from build123d import *

# Parameters (mm, degrees)
PAD_DEPTH       = 3
SKETCH001_R     = 2.125
POCKET_DEPTH    = 2.15
CHAMFER_SIZE    = 0.2
CHAMFER001_SIZE = 0.2


with BuildPart() as part:
    # Sketch → Pad (new body)
    with BuildSketch(Plane.XY):
        Polygon((4.618802, 0), (2.309401, 4), (-2.309401, 4), (-4.618802, 0), (-2.309401, -4), (2.309401, -4), (4.618802, -8), (9.237604, -8), (11.547005, -4), (9.237604, 0), align=None)
    extrude(amount=PAD_DEPTH)

    # Sketch001 → Pocket (cut)
    with BuildSketch(Plane.XY):
        Circle(SKETCH001_R)
    extrude(amount=POCKET_DEPTH, mode=Mode.SUBTRACT)

    # Chamfer
    chamfer_edges = [part.edges().sort_by_distance(p)[0] for p in [
        (3.464102, 2, 3),
        (0, 4, 3),
        (-3.464102, 2, 3),
        (-3.464102, -2, 3),
        (0, -4, 3),
        (3.464102, -6, 3),
        (6.928203, -8, 3),
        (10.392305, -6, 3),
        (10.392305, -2, 3),
        (6.928203, 0, 3),
    ]]
    chamfer(chamfer_edges, length=CHAMFER_SIZE)

    # Chamfer001
    chamfer001_edges = [part.edges().sort_by_distance(p)[0] for p in [
        (3.464102, 2, 0),
        (6.928203, 0, 0),
        (0, 4, 0),
        (10.392305, -2, 0),
        (-3.464102, 2, 0),
        (10.392305, -6, 0),
        (-3.464102, -2, 0),
        (6.928203, -8, 0),
        (0, -4, 0),
        (3.464102, -6, 0),
        (-2.125, 0, 0),
    ]]
    chamfer(chamfer001_edges, length=CHAMFER001_SIZE)


solid = part.part
For this review, take the finished solid that the model builds, in its own axes (mm). A direction names the side the tool comes from. Round coordinates to 2 decimals unless told otherwise and drop trailing zeros. Loops run counter-clockwise (first coordinate to the right, second up) from the corner with the lowest first, then second, coordinate; pieces in that order, holes last. Notation, with made-up numbers: (47.25, -36) - (62.25, -36) arc R28 cw to (62.25, -13) - close; hole circle Ø6 at (53.25, -4.5). An arc over 180 degrees is marked (long way). One line per item, written item: value. Start each with the question number.
Item 1: Take a section at D-D (y = 2.75). Give the boundary of the cut face in (x, z).
Item 2: Take a section at A-A (z = 1.3). Give the boundary of the cut face in (x, y) (3 decimals), plus the area to 3 significant figures.
Item 3: The part is to be moulded in two halves that separate along Y. For faces 3 (the flat face through (3, -2, 0)), 4 (the flat face through (10.41, -2.03, 1.48)), 5 (the flat face through (0, 0, 2.15)), 6 (the flat face through (7, -8, 1)), say which applies: +Y half, -Y half, draft (parallel to the pull), parting line (faces both ways), or undercut.
Item 4: Take a section at C-C (x = 7.5). Give the boundary of the cut face in (y, z), plus the area to 3 significant figures.
Item 5: For faces 1 (the flat face through (7, 0, 1)), 2 (the flat face through (3.448, -5.972, 1.482)), list the 3-axis set-ups (+Z, -Z, +X, -X, +Y, -Y) from which the entire face can be reached by the end or side of a thin tool; tool diameter is ignored.
Item 6: Take a section at B-B (z = 2.45). Give the boundary of the cut face in (x, y), plus the area to 3 significant figures.
Item 7: For L1, parallel to Y at x = -2.25, z = 2.1; L2, parallel to Y at x = 0, z = 0.9 (3 decimals); L3, parallel to Y at x = 6, z = 0.65, list the stretches that pass through material, from the lowest coordinate up.
Item 8: Clearance check with flat-ended pins moving along their axes: pin 1 Ø1.5 at (y, z) = (-1, 1.5) entering from -X; pin 2 Ø0.8 at (x, z) = (7.5, 1.5) entering from +Y. State where each tip first meets the part, or that it passes through.
Answer below:
1. outline: (-3.03, 0.2) - (-2.8, 0) - (2.8, 0) - (3.03, 0.2) - (3.03, 2.8) - (2.8, 3) - (-2.8, 3) - (-3.03, 2.8) - close
2. outline: (-4.619, 0) - (-2.309, -4) - (2.309, -4) - (4.619, -8) - (9.238, -8) - (11.547, -4) - (9.238, 0) - (4.619, 0) - (2.309, 4) - (-2.309, 4) - close; hole circle Ø4.25 at (0, 0)
2. area: 96.7 mm2
3. face 3: draft
3. face 4: +Y half
3. face 5: undercut
3. face 6: -Y half
4. outline: (-8, 0.2) - (-7.8, 0) - (-0.2, 0) - (0, 0.2) - (0, 2.8) - (-0.2, 3) - (-7.8, 3) - (-8, 2.8) - close
4. area: 23.9 mm2
5. face 1: +Z, -Z, +X, +Y
5. face 2: +Z, -Z, -X, -Y
6. outline: (-4.62, 0) - (-2.31, -4) - (2.31, -4) - (4.62, -8) - (9.24, -8) - (11.55, -4) - (9.24, 0) - (4.62, 0) - (2.31, 4) - (-2.31, 4) - close
6. area: 111 mm2
7. L1: y = -4 to 4
7. L2: y = -4 to -2.125, 2.125 to 4
7. L3: y = -8 to 0
8. pin 1: stops at x = -4.47
8. pin 2: stops at y = 0
